Verification items for the finished model (mm, model axes). Face numbers are marked on the shaded views. A direction names the side the tool comes from. Coordinates: 2 decimals unless noted, no trailing zeros. Write each loop counter-clockwise with the first axis right and the second up, starting at its lowest first coordinate (ties: lowest second). Pieces come first, ordered by that corner, then holes. Notation, with made-up numbers: M 1,22.25 L 50,22.25 A25 ccw 50,39.25 Z; hole C -24,61 d2. An arc over 180 degrees is marked long. Answer in a Markdown table with one row per item.
Autodesk Inventor part; units mm, degrees
ref_plane "YZ Plane" through (0, 0, 0) normal (1, 0, 0) x (0, 1, 0)
ref_plane "XZ Plane" through (0, 0, 0) normal (0, 1, 0) x (-1, 0, 0)
ref_plane "XY Plane" through (0, 0, 0) normal (0, 0, 1) x (1, 0, 0)
sketch "Sketch1" plane through (0, 0, 0) normal (0, 1, 0) x (-1, 0, 0)
  line L0 (50, 50) -> (-50, 50)
  line L1 (-50, 50) -> (-50, -50)
  line L2 (-50, -50) -> (50, -50)
  line L3 (50, -50) -> (50, 50)
  line L4 (50, 50) -> (-50, -50) construction
  line L5 (-50, 50) -> (50, -50) construction
  point P0 (0, 0)
  dimension "d0" = 100
  dimension "d1" = 100
extrude "Extrusion1" add sketch "Sketch1" along normal blind 17
sketch "Sketch2" plane through (0, 17, 0) normal (0, 1, 0) x (1, 0, 0)
  line L0 (-50, 50) -> (-50, -50)
  line L1 (50, -50) -> (50, 50)
  line L2 (-50, -45) -> (50, -45)
  line L3 (-50, -50) -> (50, -50)
  line L4 (-50, 45) -> (50, 45)
  line L5 (50, 50) -> (-50, 50)
  point P0 (0, 0)
  dimension "d4" = 5
  dimension "d5" = 5
extrude "Extrusion2" add sketch "Sketch2" along normal blind 2 contours L4 L1 L2 L0
sketch "Sketch3" plane through (0, 19, 0) normal (0, 1, 0) x (1, 0, 0)
  line L0 (-32, -40) -> (32, -40)
  line L1 (40, -32) -> (40, 32)
  line L2 (32, 40) -> (-32, 40)
  line L3 (-40, 32) -> (-40, -32)
  line L4 (-40, -40) -> (40, 40) construction
  line L5 (40, -40) -> (-40, 40) construction
  arc A0 (32, -40) -> (40, -32) centre (32, -32) ccw
  arc A1 (40, 32) -> (32, 40) centre (32, 32) ccw
  arc A2 (-32, 40) -> (-40, 32) centre (-32, 32) ccw
  arc A3 (-40, -32) -> (-32, -40) centre (-32, -32) ccw
  point P0 (0, 0)
  dimension "d8" = 80
  dimension "d9" = 80
  dimension "d10" = 8
extrude "Extrusion3" add sketch "Sketch3" along normal blind 2
sketch "Sketch4" plane through (0, 21, 0) normal (0, 1, 0) x (1, 0, 0)
  line L0 (35, -15) -> (35, 15)
  line L1 (-35, 15) -> (-35, -15)
  line L2 (-35, -15) -> (35, 15) construction
  line L3 (35, -15) -> (-35, 15) construction
  line L4 (50, -45) -> (50, 45)
  line L5 (-50, -50) -> (50, -50)
  line L6 (-15, -35) -> (15, -35)
  line L7 (15, 35) -> (-15, 35)
  line L8 (-15, -35) -> (15, 35) construction
  line L9 (15, -35) -> (-15, 35) construction
  line L10 (-15, -35) -> (-35, -15)
  line L11 (-35, 15) -> (-15, 35)
  line L12 (15, 35) -> (35, 15)
  line L13 (15, -35) -> (35, -15)
  point P0 (0, 0)
  dimension "d13" = 85
  dimension "d16" = 85
extrude "Extrusion4" add sketch "Sketch4" along normal blind 2
sketch "Sketch5" plane through (0, 23, 0) normal (0, 1, 0) x (1, 0, 0)
  circle A0 centre (0, 0) radius 25
  dimension "d19" = 50
extrude "Extrusion5" add sketch "Sketch5" along normal blind 2
sketch "Sketch6" plane through (0, 25, 0) normal (0, 1, 0) x (1, 0, 0)
  circle A0 centre (0, 0) radius 15
  dimension "d22" = 30
extrude "Extrusion6" cut sketch "Sketch6" against normal blind 4
sketch "Sketch7" plane through (0, 21, 0) normal (0, 1, 0) x (1, 0, 0)
  circle A0 centre (-32, -32) radius 1.5
  line L0 (-50, -50) -> (50, -50)
  line L1 (-50, 45) -> (-50, -45)
  circle A1 centre (-32, 32) radius 1.5
  circle A2 centre (32, -32) radius 1.5
  circle A3 centre (32, 32) radius 1.5
  point P0 (0, 0)
  dimension "d25" = 3
  dimension "d26" = 18
  dimension "d27" = 18
  dimension "d30" = 64
  dimension "d33" = 64
hole "Hole2" at (-32, 21, 32) at (-32, 21, -32) at (32, 21, -32) at (32, 21, 32) direction (0, -1, 0) diameter 3.1211 depth 9.1 tip angle 118
properties part number "A2P3"
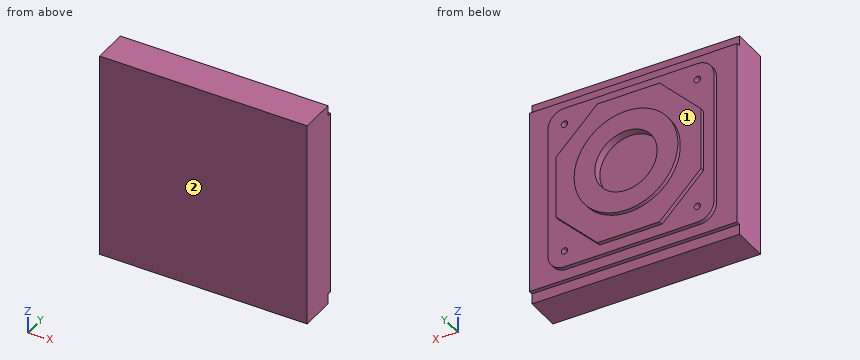
1) Thickness scan on L1, parallel to X at y = 16.25, z = 32; L2, parallel to Z at x = 0, y = 22.1; L3, parallel to Z at x = -33, y = 15.5. Record the ranges inside material, lowest first. Write a range as [from, to].
Response values:
| item | result |
|---|---|
| L1 | x = [-50, -33.56], [-30.44, 30.44], [33.56, 50] |
| L2 | z = [-35, -15], [15, 35] |
| L3 | z = [-50, -33.2], [-30.8, 30.8], [33.2, 50] |
2) Sectioned sample at A-A (z = 0). Record the cut outline in (x, y), then the cut area to 3 significant figures.
Response values:
| item | result |
|---|---|
| outline | M -50,0 L 50,0 L 50,19 L 40,19 L 40,21 L 35,21 L 35,23 L 25,23 L 25,25 L 15,25 L 15,21 L -15,21 L -15,25 L -25,25 L -25,23 L -35,23 L -35,21 L -40,21 L -40,19 L -50,19 Z |
| area | 2,180 mm² |
3) Depth check by flat-ended pin: pin 1 (1.5 mm diameter, centred on x = 11, z = 1, fed in from +Y); pin 2 (1.5 mm diameter, centred on y = 22, z = 25, fed in from +X); pin 3 (5.5 mm diameter, centred on x = -6.5, z = -48.5, fed in from +Y). Enter the tip coordinate at first touch or a pass-through.
Response values:
| item | result |
|---|---|
| pin 1 | stops at y = 21 |
| pin 2 | stops at x = 25.75 |
| pin 3 | stops at y = 17 |
4) Sectioned sample at D-D (x = -13). Record the cut outline in (y, z).
Response values:
| item | result |
|---|---|
| outline | M 0,-50 L 17,-50 L 17,-45 L 19,-45 L 19,-40 L 21,-40 L 21,-35 L 23,-35 L 23,-21.35 L 25,-21.35 L 25,-7.48 L 21,-7.48 L 21,7.48 L 25,7.48 L 25,21.35 L 23,21.35 L 23,35 L 21,35 L 21,40 L 19,40 L 19,45 L 17,45 L 17,50 L 0,50 Z |
5) Sectioned sample at C-C (x = 17.5). Record the cut outline in (y, z).
Response values:
| item | result |
|---|---|
| outline | M 0,-50 L 17,-50 L 17,-45 L 19,-45 L 19,-40 L 21,-40 L 21,-32.5 L 23,-32.5 L 23,-17.85 L 25,-17.85 L 25,17.85 L 23,17.85 L 23,32.5 L 21,32.5 L 21,40 L 19,40 L 19,45 L 17,45 L 17,50 L 0,50 Z |
6) Tool access check on the marked faces 1 and 2. Record the directions out of +Z, -Z, +X, -X, +Y, -Y that give a thin tool (end or side, any length) a straight path to the whole face; none if there is none.
Response values:
| item | result |
|---|---|
| face 1 | +Y |
| face 2 | +Z, -Z, +X, -X, -Y |
7) Sectioned sample at B-B (x = 0). Record the cut outline in (y, z), then the cut area to 3 significant figures.
Response values:
| item | result |
|---|---|
| outline | M 0,-50 L 17,-50 L 17,-45 L 19,-45 L 19,-40 L 21,-40 L 21,-35 L 23,-35 L 23,-25 L 25,-25 L 25,-15 L 21,-15 L 21,15 L 25,15 L 25,25 L 23,25 L 23,35 L 21,35 L 21,40 L 19,40 L 19,45 L 17,45 L 17,50 L 0,50 Z |
| area | 2,160 mm² |
